Here's how the part is built. I have some questions about the finished solid (model axes, mm). Coordinates: 2 decimals unless noted, no trailing zeros. Write each loop counter-clockwise with the first axis right and the second up, starting at its lowest first coordinate (ties: lowest second). Pieces come first, ordered by that corner, then holes. Notation, with made-up numbers: (89.25, 37) -> (140.25, 37) arc R22 ccw to (140.25, 48) -> close; hole circle Ø9 at (-11, 59.25). An arc over 180 degrees is marked (long way). Put each result on its own line as item: value. Start each with the question number.
Item 1: I want a section at A-A, the plane y = -1.7. List the corners of the cut face in (x, z) for me, then the cut area to 3 significant figures.
Item 2: I need wall thicknesses on line 1 (Z direction, x = 1, y = -1); line 2 (Z direction, x = 9.5, y = -2.45); line 3 (X direction, y = -1.05, z = 21). Which ranges of each line are inside material? Lowest first, please. Write a range as [from, to].
Item 3: I want a section at B-B, the plane x = 32. List the corners of the cut face in (y, z) for me, then the cut area to 3 significant figures.
Item 4: I want a section at C-C, the plane z = 28.5. List the corners of the cut face in (x, y) for me.
Item 5: For pin 1 (1.5 mm diameter, centred on x = 23, y = -1.5, fed in from +Z), with a flat end and sliding along its axis, tell me the tip position at first contact or that it passes through.
from build123d import *

# Parameters (mm, degrees)
F1_DEPTH = 2.778125
F2_R     = 2.54


with BuildPart() as f1:
    # F0 (on Front) → F1 (new body)
    with BuildSketch(Plane.XZ):
        with BuildLine():
            Line((41.148, -35.052), (41.148, 0))
            ThreePointArc((41.148, 0), (29.09603, 29.09603), (0, 41.148))
            Line((0, 41.148), (-35.052, 41.148))
            Line((-35.052, 41.148), (-35.052, -35.052))
            Line((-35.052, -35.052), (41.148, -35.052))
        make_face()
    extrude(amount=F1_DEPTH)

    # F2
    f2_edges = [f1.edges().sort_by_distance(p)[0] for p in [
        (-35.052, -1.389063, -35.052),
        (-35.052, -1.389063, 41.148),
        (41.148, -1.389063, -35.052),
    ]]
    fillet(f2_edges, radius=F2_R)


solid = f1.part
Calculated:
1. outline: (-35.05, -32.51) arc R2.54 ccw to (-32.51, -35.05) -> (38.61, -35.05) arc R2.54 ccw to (41.15, -32.51) -> (41.15, 0) arc R41.15 ccw to (0, 41.15) -> (-32.51, 41.15) arc R2.54 ccw to (-35.05, 38.61) -> close
1. area: 5,440 mm2
2. line 1: z = [-35.05, 41.14]
2. line 2: z = [-35.05, 40.04]
2. line 3: x = [-35.05, 35.39]
3. outline: (-2.78, -35.05) -> (0, -35.05) -> (0, 25.87) -> (-2.78, 25.87) -> close
3. area: 169 mm2
4. outline: (-35.05, -2.78) -> (29.68, -2.78) -> (29.68, 0) -> (-35.05, 0) -> close
5. pin 1: stops at z = 34.61
